Geometry: see drawing. Coordinates: mm, zero at the bounding-box minimum. A direction names the side the tool comes from. Round coordinates to 2 decimals unless told otherwise and drop trailing zeros. Loops run counter-clockwise (first coordinate to the right, second up) from the corner with the lowest first, then second, coordinate; pieces in that order, holes last. Notation, with made-up numbers: (43, 72.25) -> (70, 72.25) arc R12 cw to (70, 90.25) -> close; hole circle Ø8 at (85.5, -15). An arc over 180 degrees is marked (long way). Answer in a Markdown table with one row per item.
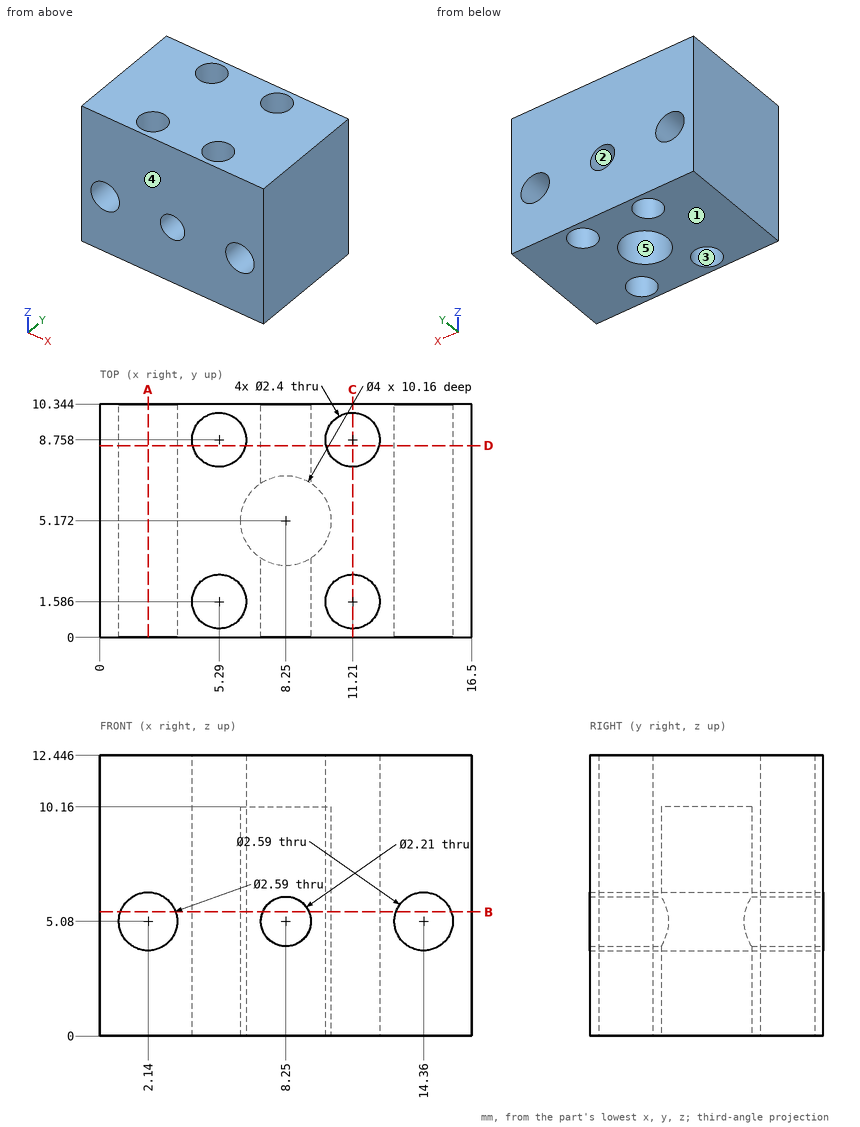
Item 1: Section query B-B, the plane z = 5.5. Output: boundary loops of the cut face in (x, y) (3 decimals).
Ans:
| item | result |
|---|---|
| outline | (0, 0) -> (0.915, 0) -> (0.915, 10.344) -> (0, 10.344) -> close; (3.365, 0) -> (7.228, 0) -> (7.228, 3.453) arc R2 cw to (7.228, 6.891) -> (7.228, 10.344) -> (3.365, 10.344) -> close; (9.272, 0) -> (13.135, 0) -> (13.135, 10.344) -> (9.272, 10.344) -> (9.272, 6.891) arc R2 cw to (9.272, 3.453) -> close; (15.585, 0) -> (16.5, 0) -> (16.5, 10.344) -> (15.585, 10.344) -> close; hole circle Ø2.4 at (5.29, 1.586); hole circle Ø2.4 at (5.29, 8.758); hole circle Ø2.4 at (11.21, 1.586); hole circle Ø2.4 at (11.21, 8.758) |
Item 2: Ray query, L1, parallel to Y at x = 5.29, z = 4.75; L2, parallel to X at y = 7.75, z = 8.5; L3, parallel to X at y = 0.5, z = 7.5. Return the intervals inside material, ascending.
Ans:
| item | result |
|---|---|
| L1 | 0 to 0.39, 2.79 to 7.56, 9.96 to 10.34 |
| L2 | 0 to 4.64, 5.94 to 10.56, 11.86 to 16.5 |
| L3 | 0 to 4.78, 5.8 to 10.7, 11.72 to 16.5 |
Item 3: Section query A-A, the plane x = 2.14. Output: boundary loops of the cut face in (y, z) (3 decimals), and give its area (3 significant figures).
Ans:
| item | result |
|---|---|
| outline | (0, 0) -> (10.344, 0) -> (10.344, 3.785) -> (0, 3.785) -> close; (0, 6.375) -> (10.344, 6.375) -> (10.344, 12.446) -> (0, 12.446) -> close |
| area | 102 mm2 |
Item 4: Section query C-C, the plane x = 11.21. Output: boundary loops of the cut face in (y, z), and give its area (3 significant figures).
Ans:
| item | result |
|---|---|
| outline | (0, 0) -> (0.39, 0) -> (0.39, 12.45) -> (0, 12.45) -> close; (2.79, 0) -> (7.56, 0) -> (7.56, 12.45) -> (2.79, 12.45) -> close; (9.96, 0) -> (10.34, 0) -> (10.34, 12.45) -> (9.96, 12.45) -> close |
| area | 69.0 mm2 |
Item 5: First-contact query: P1, Ø3, axis at x = 11.21, y = 1.586, coming from the +Z side. Flat tip, straight axial feed; report the tip coordinate or a pass-through.
Ans:
| item | result |
|---|---|
| P1 | z = 12.45 |
Item 6: Mould query, pull axis Z, two halves, no side actions, for the marked faces 1, 2 and 3. Classes: released by +Z, released by -Z, zero draft, split by the parting line, or undercut.
Ans:
| item | result |
|---|---|
| face 1 | released by -Z |
| face 2 | undercut |
| face 3 | zero draft |
Item 7: Set-up query: the marked faces 4 and 5. Return all of +Z, -Z, +X, -X, +Y, -Y with unobstructed straight access to the full face (end or side cutting, diameter ignored); none if empty.
Ans:
| item | result |
|---|---|
| face 4 | +Z, -Z, +X, -X, -Y |
| face 5 | -Z |
Item 8: Section query D-D, the plane y = 8.5. Output: boundary loops of the cut face in (x, z) (3 decimals).
Ans:
| item | result |
|---|---|
| outline | (0, 0) -> (4.118, 0) -> (4.118, 12.446) -> (0, 12.446) -> close; (6.462, 0) -> (10.038, 0) -> (10.038, 12.446) -> (6.462, 12.446) -> close; (12.382, 0) -> (16.5, 0) -> (16.5, 12.446) -> (12.382, 12.446) -> close; hole circle Ø2.59 at (2.14, 5.08); hole circle Ø2.21 at (8.25, 5.08); hole circle Ø2.59 at (14.36, 5.08) |
